The figure shows three views and two pictorial views of one solid part (mm, origin at its lowest corner). Answer the questions. A direction names the side the tool comes from. Give positions to 0.01 mm unless a question says otherwise; leave off trailing zeros. Order: outer loops, then holes, each group sorted by start corner. A loop starts at its lowest first (then second) coordinate and runs counter-clockwise, first axis right, second up. Notation, with made-up numbers: M 0.5,28.5 L 15.5,28.5 A6 ccw 15.5,33.5 Z; hole C 24,-40 d5. An arc over 180 degrees is marked long. Write item = value, one per line. Start each with the question number.
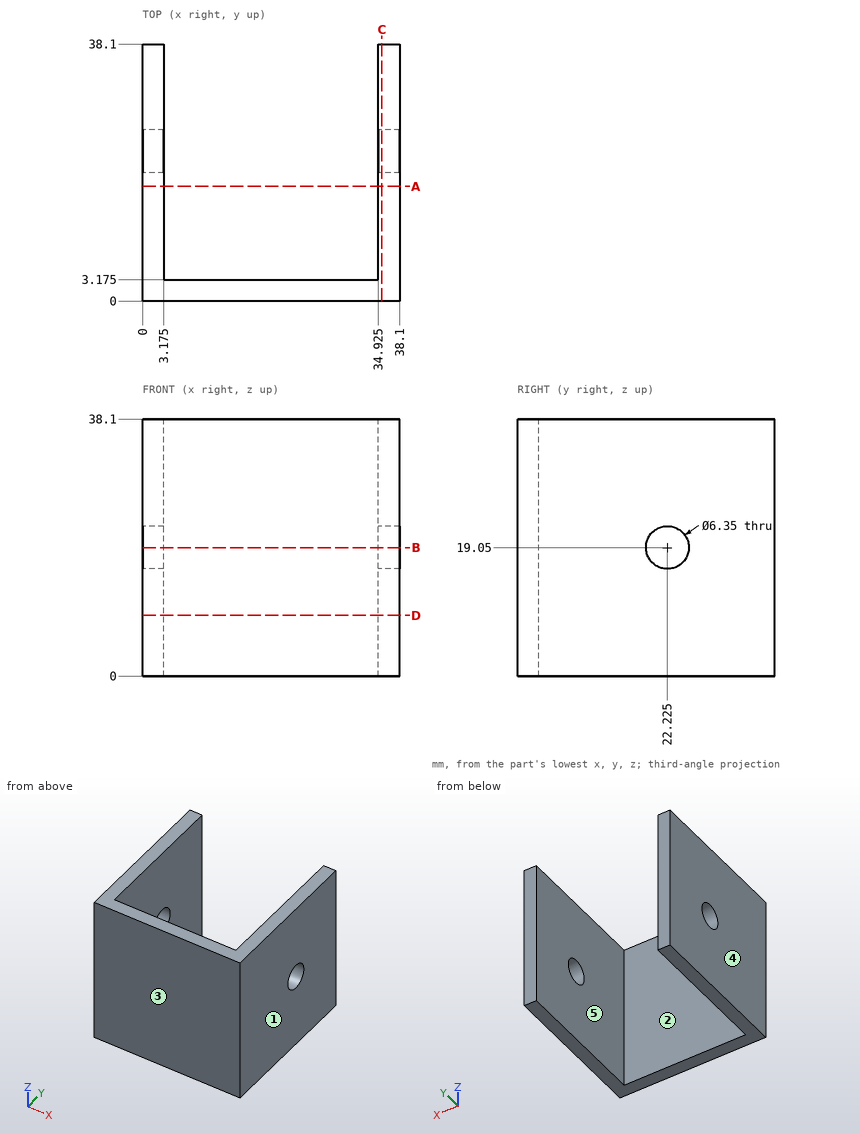
1) Find section C-C on x = 35.5. Determine the outline of the cut face in (y, z) (3 decimals), plus the area to 3 significant figures.
2) Each of these flat-tipped pins is pushed along its axis until it touches: P1, Ø2, axis at x = 4.5, y = 24.5, coming from the +Z side; P2, Ø8, axis at x = 28.5, z = 10, coming from the +Y side (3 decimals). Where does it stop, or does it pass through?
3) Find section B-B on z = 19.05. Determine the outline of the cut face in (x, y) (3 decimals), plus the area to 3 significant figures.
4) For the marked faces 1 and 2, determine the directions among +Z, -Z, +X, -X, +Y, -Y from which every point of the face is accessible in a straight line to the end or side of a thin tool.
5) Find section A-A on y = 17. Determine the outline of the cut face in (x, z) (3 decimals), plus the area to 3 significant figures.
6) For a pull along X with two mould halves and no side action, classify the marked faces 3, 4 and 5 as pulls with the +X half, pulls with the -X half, needs draft (parallel to the pull), parting line crosses it, or undercut.
7) Find section D-D on z = 9. Determine the outline of the cut face in (x, y) (3 decimals), plus the area to 3 significant figures.
8) Find the intervals of material crossed by probe 1 along Y at (x, z) = (1, 19); probe 2 along X at (y, z) = (29, 16) (3 decimals); probe 3 along Y at (x, z) = (26, 16) (3 decimals), in increasing order. Write a range as [from, to].
Numbers:
q1.outline = M 0,0 L 38.1,0 L 38.1,38.1 L 0,38.1 Z; hole C 22.225,19.05 d6.35
q1.area = 1,420 mm2
q2.P1 = through
q2.P2 = 3.175
q3.outline = M 0,0 L 38.1,0 L 38.1,19.05 L 34.925,19.05 L 34.925,3.175 L 3.175,3.175 L 3.175,19.05 L 0,19.05 Z; M 0,25.4 L 3.175,25.4 L 3.175,38.1 L 0,38.1 Z; M 34.925,25.4 L 38.1,25.4 L 38.1,38.1 L 34.925,38.1 Z
q3.area = 302 mm2
q4.face_1 = +Z, -Z, +X, +Y, -Y
q4.face_2 = +Z, -Z, +Y
q5.outline = M 0,0 L 3.175,0 L 3.175,38.1 L 0,38.1 Z; M 34.925,0 L 38.1,0 L 38.1,38.1 L 34.925,38.1 Z
q5.area = 242 mm2
q6.face_3 = needs draft
q6.face_4 = pulls with the -X half
q6.face_5 = undercut
q7.outline = M 0,0 L 38.1,0 L 38.1,38.1 L 34.925,38.1 L 34.925,3.175 L 3.175,3.175 L 3.175,38.1 L 0,38.1 Z
q7.area = 343 mm2
q8.probe_1 = [0, 19.05], [25.4, 38.1]
q8.probe_2 = [0, 3.175], [34.925, 38.1]
q8.probe_3 = [0, 3.175]
